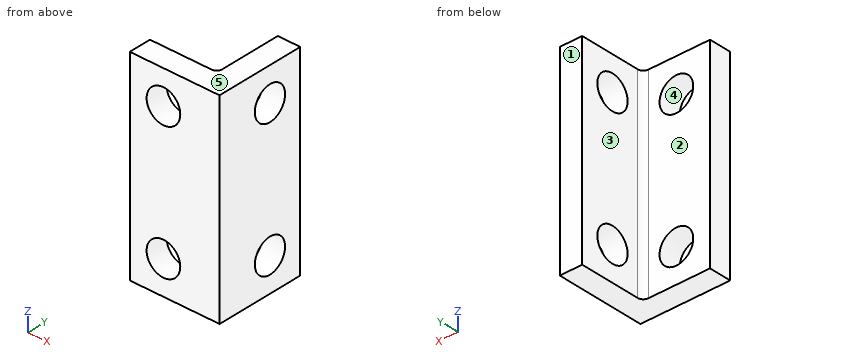
```python
from build123d import *

# Parameters (mm, degrees)
BOSS_EXTRUDE1_DEPTH     = 18
CUT_EXTRUDE1_DEPTH      = 22.260291625
CUT_EXTRUDE1_DEPTH_BACK = 22.260291625
SKETCH2_R               = 1.5
CUT_EXTRUDE2_DEPTH      = 22.260291625
CUT_EXTRUDE2_DEPTH_BACK = 22.260291625
SKETCH3_R               = 1.5
FILLET1_R               = 0.5


with BuildPart() as part:
    # Sketch1 → Boss-Extrude1 (new body)
    with BuildSketch(Plane.XY):
        Polygon((0, 0), (-8, 0), (-8, 2), (-2, 2), (-2, 8), (0, 8), align=None)
    extrude(amount=BOSS_EXTRUDE1_DEPTH)

    # Sketch2 → Cut-Extrude1 (cut, two sides: drawn at the far end of the back side and taken through both)
    with BuildSketch(Plane(origin=(0, 0, 0), x_dir=(0, 0, -1), z_dir=(1, 0, 0)).offset(-CUT_EXTRUDE1_DEPTH_BACK)):
        with Locations(Location((-15, 5, 0), (0, 0, 90))):
            Circle(SKETCH2_R)
        with Locations(Location((-3, 5, 0), (0, 0, 90))):
            Circle(SKETCH2_R)
    extrude(amount=CUT_EXTRUDE1_DEPTH + CUT_EXTRUDE1_DEPTH_BACK, mode=Mode.SUBTRACT)

    # Sketch3 → Cut-Extrude2 (cut, two sides: drawn at the far end of the back side and taken through both)
    with BuildSketch(Plane.XZ.offset(-CUT_EXTRUDE2_DEPTH_BACK)):
        with Locations((-5, 15)):
            Circle(SKETCH3_R)
        with Locations((-5, 3)):
            Circle(SKETCH3_R)
    extrude(amount=CUT_EXTRUDE2_DEPTH + CUT_EXTRUDE2_DEPTH_BACK, mode=Mode.SUBTRACT)

    # Fillet1
    fillet1_edges = [part.edges().sort_by_distance(p)[0] for p in [
        (-2, 2, 9),
    ]]
    fillet(fillet1_edges, radius=FILLET1_R)


solid = part.part
```
The listing builds one solid part. Answer for the finished solid, in the listing's coordinates (mm). Face numbers are marked on the shaded views. A direction names the side the tool comes from. Coordinates: 2 decimals unless noted, no trailing zeros. Write each loop counter-clockwise with the first axis right and the second up, starting at its lowest first coordinate (ties: lowest second). Pieces come first, ordered by that corner, then holes. Notation, with made-up numbers: (62.25, 46) - (112.25, 46) arc R28 ccw to (112.25, 82) - close; hole circle Ø7 at (-12, -27.75). An arc over 180 degrees is marked (long way). Return JSON: item names as keys, results as strings. Group by question number.
1. A cutting plane is placed at D-D, the plane z = 9.25. Determine the outline of the cut face in (x, y), plus the area to 3 significant figures.
2. Given pin 1 (4 mm diameter, centred on y = 5, z = 3, fed in from -X); pin 2 (4.5 mm diameter, centred on x = -6.5, z = 7.5, fed in from +Y), each flat-ended and moving along its own axis, determine where each tip first touches the part or whether it passes through.
3. Determine the mould class of the marked faces 3, 4 and 5 for opening direction X: released by +X, released by -X, zero draft, split by the parting line, or undercut.
4. A cutting plane is placed at A-A, the plane y = 5. Determine the outline of the cut face in (x, z).
5. Which of the six approach directions +Z, -Z, +X, -X, +Y, -Y give full straight-line access (tool end or side, diameter ignored) to the marked faces 1 and 2?
6. A cutting plane is placed at C-C, the plane x = -5. Determine the outline of the cut face in (y, z), plus the area to 3 significant figures.
7. A cutting plane is placed at B-B, the plane z = 15. Determine the outline of the cut face in (x, y), plus the area to 3 significant figures.
8. Straight lines are drawn through the part: L1, parallel to Z at x = -1.3, y = 5; L2, parallel to Y at x = -1.1, z = 3; L3, parallel to X at y = 0.85, z = 3. For each, find the intervals that lie inside material, in ascending order.
Ans:
{
 "1": {"outline": "(-8, 0) - (0, 0) - (0, 8) - (-2, 8) - (-2, 2.5) arc R0.5 cw to (-2.5, 2) - (-8, 2) - close", "area": "28.1 mm²"},
 "2": {"pin 1": "x = -2", "pin 2": "y = 2"},
 "3": {"face 3": "released by -X", "face 4": "undercut", "face 5": "zero draft"},
 "4": {"outline": "(-2, 0) - (0, 0) - (0, 1.5) - (-2, 1.5) - close; (-2, 4.5) - (0, 4.5) - (0, 13.5) - (-2, 13.5) - close; (-2, 16.5) - (0, 16.5) - (0, 18) - (-2, 18) - close"},
 "5": {"face 1": "+Z, -Z, +X, -X, +Y", "face 2": "+Z, -Z, -X, +Y"},
 "6": {"outline": "(0, 0) - (2, 0) - (2, 1.5) - (0, 1.5) - close; (0, 4.5) - (2, 4.5) - (2, 13.5) - (0, 13.5) - close; (0, 16.5) - (2, 16.5) - (2, 18) - (0, 18) - close", "area": "24.0 mm²"},
 "7": {"outline": "(-8, 0) - (-6.5, 0) - (-6.5, 2) - (-8, 2) - close; (-3.5, 0) - (0, 0) - (0, 3.5) - (-2, 3.5) - (-2, 2.5) arc R0.5 cw to (-2.5, 2) - (-3.5, 2) - close; (-2, 6.5) - (0, 6.5) - (0, 8) - (-2, 8) - close", "area": "16.1 mm²"},
 "8": {"L1": "0 to 1.5, 4.5 to 13.5, 16.5 to 18", "L2": "0 to 3.5, 6.5 to 8", "L3": "-8 to -6.5, -3.5 to 0"}
}
